The model under review builds one solid part; all positions refer to its coordinate system, in mm. Give positions to 0.01 mm unless a question says otherwise; leave off trailing zeros. Order: outer loops, then holes, each group sorted by start corner. A loop starts at its lowest first (then second) coordinate and runs counter-clockwise, first axis right, second up. Notation, with made-up numbers: (-12.75, 32) - (-5.75, 32) arc R19 ccw to (-5.75, 65) - close; hole circle Ø5 at (-35.75, 11). An arc over 180 degrees is marked (long way). Answer as CSV lines item,"result". Start each with the question number.
from build123d import *

# Parameters (mm, degrees)
SKETCH1_W                = 45
SKETCH1_H                = 28
BOSS_EXTRUDE1_DEPTH      = 30
BOSS_EXTRUDE2_DEPTH      = 5
BOSS_EXTRUDE2_DEPTH_BACK = 5


with BuildPart() as part:
    # Sketch1 → Boss-Extrude1 (new body)
    with BuildSketch(Plane(origin=(0, 0, 0), x_dir=(1, 0, 0), z_dir=(0, 1, 0))):
        Rectangle(SKETCH1_W, SKETCH1_H)
    extrude(amount=BOSS_EXTRUDE1_DEPTH)

    # Sketch2 → Boss-Extrude2 (add, two sides: drawn at the far end of the back side and taken through both)
    with BuildSketch(Plane.XY.offset(-BOSS_EXTRUDE2_DEPTH_BACK)):
        Polygon((22.5, 4), (25.900415076, 4), (35.114670864, 29.315959713), (33.235285622, 30), (24.5, 6), (22.5, 6), align=None)
    extrude(amount=BOSS_EXTRUDE2_DEPTH + BOSS_EXTRUDE2_DEPTH_BACK)


solid = part.part
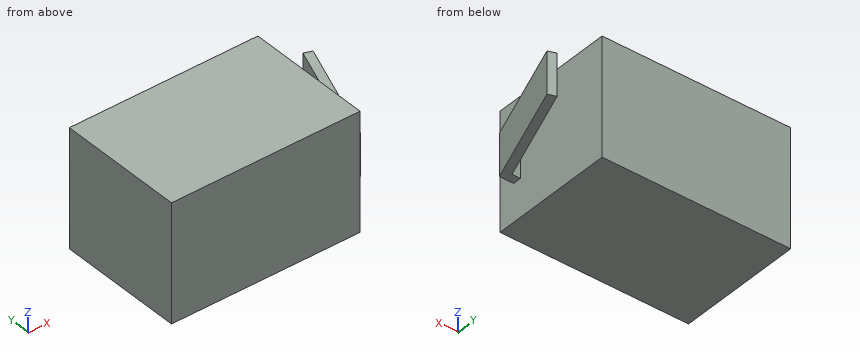
Item 1: For line 1 along X through (y, z) = (9.5, 6); line 2 along X through (y, z) = (16.5, 1.5); line 3 along X through (y, z) = (10, 4), list the stretches that pass through material, from the lowest coordinate up.
Item 2: Take a section at A-A on y = 19.5. Write out the cut boundary in (x, z), and give its area (3 significant figures).
Item 3: Clearance check with flat-ended pins moving along their axes: pin 1 (6.5 mm diameter, centred on x = 26.5, y = 12.5, fed in from -Z); pin 2 (1.5 mm diameter, centred on y = 22, z = -7.5, fed in from +X); pin 3 (10 mm diameter, centred on x = 28, y = 18.5, fed in from +Z). State where each tip first meets the part, or that it passes through.
Item 4: Take a section at B-B on z = -4.25. Write out the cut boundary in (x, y).
Item 5: Take a section at C-C on y = 5. Write out the cut boundary in (x, z), and give its area (3 significant figures).
Item 6: Take a section at D-D on z = 10.75. Write out the cut boundary in (x, y).
Data:
1,line 1,"x = -22.5 to 22.5"
1,line 2,"x = -22.5 to 22.5, 28.32 to 30.45"
1,line 3,"x = -22.5 to 22.5, 25.96 to 28.08"
2,outline,"(-22.5, -14) - (22.5, -14) - (22.5, 14) - (-22.5, 14) - close; (29.41, -5) - (31.54, -5) - (31.54, 5) - (29.41, 5) - close"
2,area,"1,280 mm^2"
3,pin 1,"stops at z = -5"
3,pin 2,"stops at x = 22.5"
3,pin 3,"stops at z = 5"
4,outline,"(-22.5, 0) - (22.5, 0) - (22.5, 4) - (25.9, 4) - (35.11, 29.32) - (33.24, 30) - (24.5, 6) - (22.5, 6) - (22.5, 30) - (-22.5, 30) - close"
5,outline,"(-22.5, -14) - (22.5, -14) - (22.5, -5) - (26.26, -5) - (26.26, 5) - (22.5, 5) - (22.5, 14) - (-22.5, 14) - close"
5,area,"1,300 mm^2"
6,outline,"(-22.5, 0) - (22.5, 0) - (22.5, 30) - (-22.5, 30) - close"
